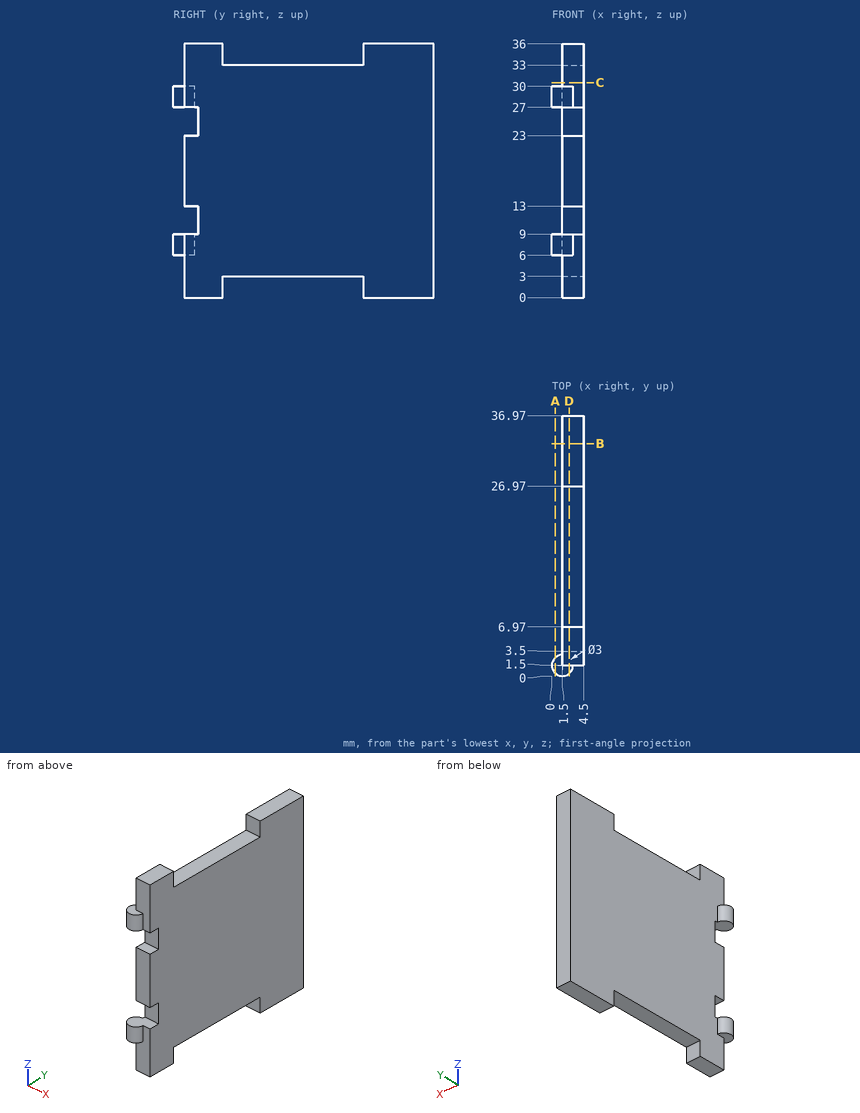
Part print with two shaded views. Sizes in mm from the minimum x, y, z corner. Give positions to 0.01 mm unless a question says otherwise; leave off trailing zeros. Order: outer loops, then holes, each group sorted by start corner. A loop starts at its lowest first (then second) coordinate and runs counter-clockwise, first axis right, second up. Notation, with made-up numbers: M -39.75,31.25 L -10.75,31.25 A16 cw -10.75,60.25 Z; hole C -40,-19 d7. An arc over 180 degrees is marked long. Write item = value, one per line.
Q1. Cut at C-C, the plane z = 30.5. List the corners of the cut face in (x, y).
Derived:
outline = M 1.5,1.5 L 4.5,1.5 L 4.5,36.97 L 1.5,36.97 Z
Q2. Cut at B-B, the plane y = 33. List the corners of the cut face in (x, z), then the cut area to 3 significant figures.
Derived:
outline = M 1.5,0 L 4.5,0 L 4.5,36 L 1.5,36 Z
area = 108 mm2
Q3. Flat gauge pins, fed straight in: pin 1 (1 mm diameter, centred on y = 25.5, z = 10, fed in from -X); pin 2 (1 mm diameter, centred on x = 1.5, y = 16.5, fed in from -Z); pin 3 (0.9 mm diameter, centred on x = 1.5, y = 1, fed in from +Z); pin 4 (0.9 mm diameter, centred on x = 2, y = 2, fed in from -Z). Where does each tip first touch, or does it go through?
Derived:
pin_1 = 1.5
pin_2 = 3
pin_3 = 30
pin_4 = 0
Q4. Drill centre lines: line 1 (Y direction, x = 1.85, z = 2.5); line 2 (Y direction, x = 3.8, z = 15); line 3 (Y direction, x = 1.75, z = 26.5). Where is each one in solid material? Low to high. Write a range as [from, to].
Derived:
line_1 = [1.5, 6.97], [26.97, 36.97]
line_2 = [1.5, 36.97]
line_3 = [3.5, 36.97]
Q5. Cut at D-D, the plane x = 2.45. List the corners of the cut face in (y, z), then the cut area to 3 significant figures.
Derived:
outline = M 0.34,6 L 1.5,6 L 1.5,0 L 6.97,0 L 6.97,3 L 26.97,3 L 26.97,0 L 36.97,0 L 36.97,36 L 26.97,36 L 26.97,33 L 6.97,33 L 6.97,36 L 1.5,36 L 1.5,30 L 0.34,30 L 0.34,27 L 3.5,27 L 3.5,23 L 1.5,23 L 1.5,13 L 3.5,13 L 3.5,9 L 0.34,9 Z
area = 1,150 mm2
Q6. Cut at A-A, the plane x = 0.5. List the corners of the cut face in (y, z), then the cut area to 3 significant figures.
Derived:
outline = M 0.38,6 L 2.62,6 L 2.62,9 L 0.38,9 Z; M 0.38,27 L 2.62,27 L 2.62,30 L 0.38,30 Z
area = 13.4 mm2
